Geometry check sheet. Reference: drawing and pictorial views, mm from the part's lowest x, y, z. Give positions to 0.01 mm unless a question says otherwise; leave off trailing zeros. Loops run counter-clockwise (first coordinate to the right, second up) from the corner with the lowest first, then second, coordinate; pieces in that order, holes last. Notation, with made-up numbers: M 26.5,28 L 46.5,28 A16 ccw 46.5,34 Z; hole C 85.25,55 d7. An arc over 180 degrees is marked long. Use CSV: the item, a comma, the result in double quotes.
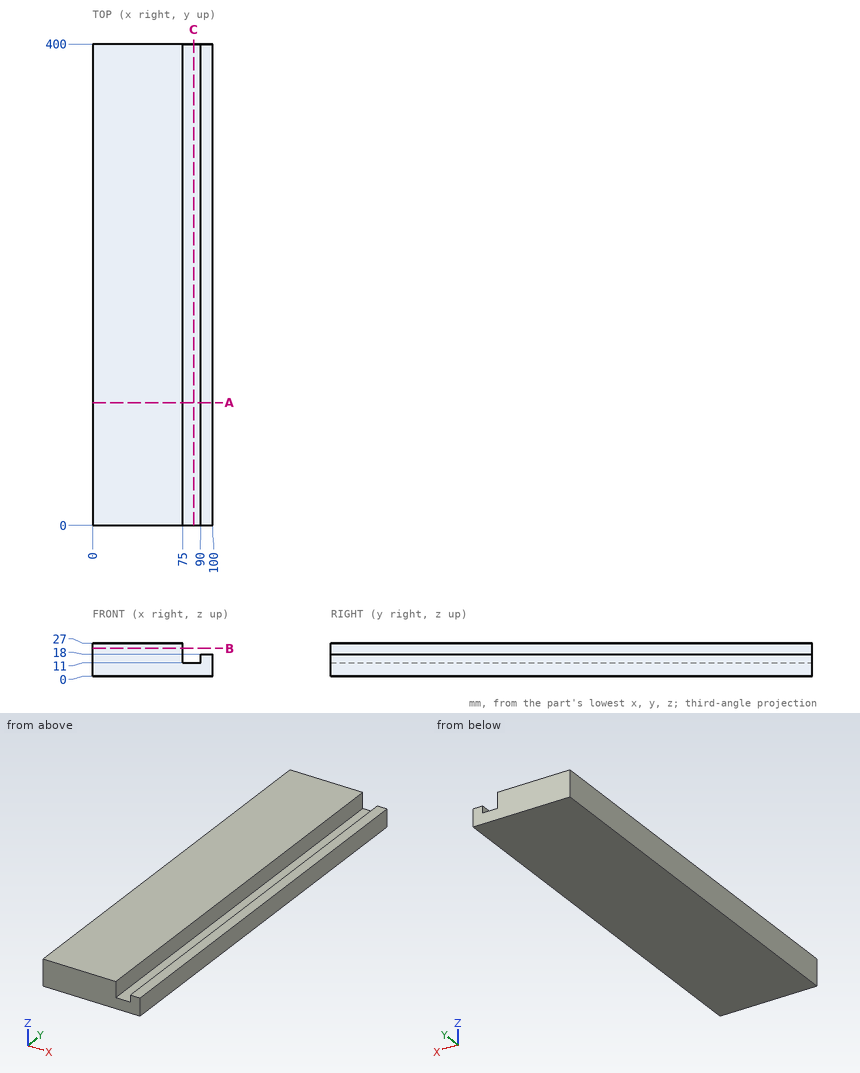
(1) Section check C-C on x = 84. Record the cut outline in (y, z).
Calculated:
outline,"M 0,0 L 400,0 L 400,11 L 0,11 Z"
(2) Section check B-B on z = 23. Record the cut outline in (x, y), plus the area to 3 significant figures.
Calculated:
outline,"M 0,0 L 75,0 L 75,400 L 0,400 Z"
area,"30,000 mm²"
(3) Section check A-A on y = 102. Record the cut outline in (x, z).
Calculated:
outline,"M 0,0 L 100,0 L 100,18 L 90,18 L 90,11 L 75,11 L 75,27 L 0,27 Z"
(4) Depth check by flat-ended pin: pin 1 Ø3 at (y, z) = (287, 21) entering from +X; pin 2 Ø16.5 at (x, y) = (84, 264.5) entering from +Z. Enter the tip coordinate at first touch or a pass-through.
Calculated:
pin 1,"stops at x = 75"
pin 2,"stops at z = 18"
(5) Scan lines: L1, parallel to X at y = 88.5, z = 13; L2, parallel to Z at x = 87.5, y = 242.5; L3, parallel to X at y = 262, z = 23.75. Record each from-to range of solid material in increasing order. Write a range as from..to.
Calculated:
L1,"x = 0..75, 90..100"
L2,"z = 0..11"
L3,"x = 0..75"
